For this review, take the finished solid that the model builds, in its own axes (mm). A direction names the side the tool comes from. Round coordinates to 2 decimals unless told otherwise and drop trailing zeros. Order: outer loops, then holes, each group sorted by start corner. A loop starts at its lowest first (then second) coordinate and runs counter-clockwise, first axis right, second up. Notation, with made-up numbers: M -18.75,-8.75 L -10.75,-8.75 A14 ccw -10.75,2.25 Z; hole C 27,67.5 d11. An arc over 180 degrees is marked long. Use a Markdown table: item, result.
from build123d import *

# Parameters (mm, degrees)
SKETCH1_R                                           = 32
SKETCH1_R_2                                         = 15
BOSS_EXTRUDE1_DEPTH                                 = 6
CBORE_FOR_M4_HEX_SOCKET_HEAD_CAP_SCREW2_D           = 4.3
CBORE_FOR_M4_HEX_SOCKET_HEAD_CAP_SCREW2_DEPTH       = 11.94
CBORE_FOR_M4_HEX_SOCKET_HEAD_CAP_SCREW2_CBORE_D     = 8
CBORE_FOR_M4_HEX_SOCKET_HEAD_CAP_SCREW2_CBORE_DEPTH = 4.4
CBORE_FOR_M4_HEX_SOCKET_HEAD_CAP_SCREW2_TIP         = 1.291850331
SKETCH7_R                                           = 2
CUT_EXTRUDE1_DEPTH                                  = 44.5
SKETCH8_R                                           = 2
CUT_EXTRUDE2_DEPTH                                  = 44.5
CUT_EXTRUDE3_START                                  = -10
CUT_EXTRUDE3_DEPTH                                  = 10


with BuildPart() as part:
    # Sketch1 → Boss-Extrude1 (new body)
    with BuildSketch(Plane(origin=(0, 0, 0), x_dir=(1, 0, 0), z_dir=(0, 1, 0))):
        with Locations(Location((0, 0, 0), (0, 0, 270))):
            Circle(SKETCH1_R)
        with Locations(Location((0, 0, 0), (0, 0, 270))):
            Circle(SKETCH1_R_2, mode=Mode.SUBTRACT)
    extrude(amount=BOSS_EXTRUDE1_DEPTH)

    # CBORE for M4 Hex Socket Head Cap Screw2
    with Locations(Plane(origin=(0, 6, 0), x_dir=(1, 0, 0), z_dir=(0, 1, 0))):
        with Locations((19.091883092, 19.091883092), (19.091883092, -19.091883092), (-19.091883092, -19.091883092), (-19.091883092, 19.091883092)):
            CounterBoreHole(CBORE_FOR_M4_HEX_SOCKET_HEAD_CAP_SCREW2_D / 2, CBORE_FOR_M4_HEX_SOCKET_HEAD_CAP_SCREW2_CBORE_D / 2, CBORE_FOR_M4_HEX_SOCKET_HEAD_CAP_SCREW2_CBORE_DEPTH, depth=CBORE_FOR_M4_HEX_SOCKET_HEAD_CAP_SCREW2_DEPTH)
            with Locations((0, 0, -(CBORE_FOR_M4_HEX_SOCKET_HEAD_CAP_SCREW2_DEPTH + CBORE_FOR_M4_HEX_SOCKET_HEAD_CAP_SCREW2_TIP / 2))):  # 118° drill point
                Cone(0, CBORE_FOR_M4_HEX_SOCKET_HEAD_CAP_SCREW2_D / 2, CBORE_FOR_M4_HEX_SOCKET_HEAD_CAP_SCREW2_TIP, mode=Mode.SUBTRACT)

    # Sketch7 → Cut-Extrude1 (cut)
    with BuildSketch(Plane(origin=(0, 0, 0), x_dir=(0, 0, -1), z_dir=(1, 0, 0))):
        with Locations(Location((0, 3, 0), (0, 0, 180))):
            Circle(SKETCH7_R)
    extrude(amount=CUT_EXTRUDE1_DEPTH, mode=Mode.SUBTRACT)

    # Sketch8 → Cut-Extrude2 (cut)
    with BuildSketch(Plane.XY):
        with Locations(Location((0, 3, 0), (0, 0, 90))):
            Circle(SKETCH8_R)
    extrude(amount=-CUT_EXTRUDE2_DEPTH, mode=Mode.SUBTRACT)

    # Sketch9 → Cut-Extrude3 (cut)
    with BuildSketch(Plane(origin=(0, 6, 0), x_dir=(1, 0, 0), z_dir=(0, 1, 0)).offset(CUT_EXTRUDE3_START)):
        with BuildLine():
            Line((-27.5, 16.363068172), (-27.5, -16.363068172))
            ThreePointArc((-27.5, -16.363068172), (-32, 0), (-27.5, 16.363068172))
        make_face()
        with BuildLine():
            Line((27.5, -16.363068172), (27.5, 16.363068172))
            ThreePointArc((27.5, 16.363068172), (32, 0), (27.5, -16.363068172))
        make_face()
    extrude(amount=CUT_EXTRUDE3_DEPTH, mode=Mode.SUBTRACT)


solid = part.part
Q1. Add section A-A (x = 0). Write out the cut boundary in (y, z).
Determined:
| item | result |
|---|---|
| outline | M 0,-32 L 1,-32 L 1,-15 L 0,-15 Z; M 0,15 L 6,15 L 6,32 L 0,32 Z; M 5,-32 L 6,-32 L 6,-15 L 5,-15 Z |
Q2. Clearance check with flat-ended pins moving along their axes: pin 1 (6.5 mm diameter, centred on x = 19.09, z = 19.09, fed in from +Y); pin 2 (6 mm diameter, centred on x = 20, z = 5, fed in from -Y). State where each tip first meets the part, or that it passes through.
Determined:
| item | result |
|---|---|
| pin 1 | stops at y = 1.6 |
| pin 2 | stops at y = 0 |
Q3. Add section D-D (z = -11). Write out the cut boundary in (x, y), then the cut area to 3 significant figures.
Determined:
| item | result |
|---|---|
| outline | M -27.5,0 L -10.2,0 L -10.2,6 L -27.5,6 Z; M 10.2,0 L 27.5,0 L 27.5,6 L 10.2,6 Z |
| area | 208 mm^2 |
Q4. Add section B-B (z = 0). Write out the cut boundary in (x, y), then the cut area to 3 significant figures.
Determined:
| item | result |
|---|---|
| outline | M -27.5,0 L -15,0 L -15,6 L -27.5,6 Z; M 15,0 L 27.5,0 L 27.5,1 L 15,1 Z; M 15,5 L 27.5,5 L 27.5,6 L 15,6 Z |
| area | 100 mm^2 |
Q5. Machinability: for faces 1 (the cylindrical face through (2, 3, -23)), 2 (the flat face through (-17, 1.6, 21)), 3 (the cylindrical face through (-17.39, 0.79, -17.78)), which of the approach directions +Z, -Z, +X, -X, +Y, -Y give a long, thin tool a straight path to every point of the face, cutting with its end or side? Answer none if there is none.
Determined:
| item | result |
|---|---|
| face 1 | -Z |
| face 2 | +Y |
| face 3 | +Y, -Y |
Q6. Add section C-C (y = 3). Write out the cut boundary in (x, z), then the cut area to 3 significant figures.
Determined:
| item | result |
|---|---|
| outline | M -27.5,-16.36 A32 ccw -2,-31.94 L -2,-14.87 A15 cw long 14.87,2 L 27.5,2 L 27.5,16.36 A32 ccw -27.5,16.36 Z; M 2,-31.94 A32 ccw 27.5,-16.36 L 27.5,-2 L 14.87,-2 A15 cw 2,-14.87 Z; hole C -19.09,-19.09 d8; hole C -19.09,19.09 d8; hole C 19.09,-19.09 d8; hole C 19.09,19.09 d8 |
| area | 1,990 mm^2 |
Q7. Draft analysis for pull direction X (two halves, no side actions). For faces 4 (the flat face through (-17, 1.6, -17)), 5 (the flat face through (-6, 0, -15)), 6 (the flat face through (27.5, 0.3, 0.2)), state which applies: pulls with the +X half, pulls with the -X half, needs draft (parallel to the pull), parting line crosses it, or undercut.
Determined:
| item | result |
|---|---|
| face 4 | undercut |
| face 5 | needs draft |
| face 6 | pulls with the +X half |
Q8. Wall thickness on line 1 along Z through (x, y) = (-19.5, 4.5); line 2 along X through (y, z) = (4.5, 15.5); line 3 along Z through (x, y) = (-20, 2.75): over which ranges is each line inside the solid? List them lowest first. Write a range as [from, to].
Determined:
| item | result |
|---|---|
| line 1 | z = [-25.37, -23.07], [-15.11, 15.11], [23.07, 25.37] |
| line 2 | x = [-27.5, -20.85], [-17.33, 17.33], [20.85, 27.5] |
| line 3 | z = [-24.98, -22.99], [-15.2, 15.2], [22.99, 24.98] |
